from build123d import *

# Parameters (mm, degrees)
SKETCH1_W           = 9
SKETCH1_H           = 9
BOSS_EXTRUDE1_DEPTH = 3
SKETCH2_W           = 2.95
SKETCH2_H           = 6
BOSS_EXTRUDE2_DEPTH = 6.1
FILLET1_R           = 3
SKETCH3_R           = 0.975
CUT_EXTRUDE1_DEPTH  = 11.1
CUT_EXTRUDE3_DEPTH  = 21.1
BOSS_EXTRUDE3_START = 4
SKETCH5_R           = 3
BOSS_EXTRUDE3_DEPTH = 4
SKETCH8_R           = 1.55
CUT_EXTRUDE4_DEPTH  = 3
CUT_EXTRUDE5_DEPTH  = 0.5
SKETCH10_W          = 9
SKETCH10_H          = 3
BOSS_EXTRUDE4_DEPTH = 4
SKETCH11_R          = 1
CUT_EXTRUDE6_DEPTH  = 4
CUT_EXTRUDE7_DEPTH  = 4


with BuildPart() as part:
    # Sketch1 → Boss-Extrude1 (new body)
    with BuildSketch(Plane(origin=(0, 0, 0), x_dir=(1, 0, 0), z_dir=(0, 1, 0))):
        with Locations((4.5, 4.5)):
            Rectangle(SKETCH1_W, SKETCH1_H)
    extrude(amount=BOSS_EXTRUDE1_DEPTH)

    # Sketch2 → Boss-Extrude2 (add)
    with BuildSketch(Plane(origin=(0, 0, -9), x_dir=(-1, 0, 0), z_dir=(0, 0, -1))):
        with Locations((-7.525, 1.5)):
            Rectangle(SKETCH2_W, SKETCH2_H)
        with Locations((-1.475, 1.5)):
            Rectangle(SKETCH2_W, SKETCH2_H)
    extrude(amount=BOSS_EXTRUDE2_DEPTH)

    # Fillet1
    fillet1_edges = [part.edges().sort_by_distance(p)[0] for p in [
        (1.475, 4.5, -15.1),
        (1.475, -1.5, -15.1),
        (7.525, -1.5, -15.1),
        (7.525, 4.5, -15.1),
    ]]
    fillet(fillet1_edges, radius=FILLET1_R - 0.0001)  # a hair under: the kernel refuses the full size

    # Sketch3 → Cut-Extrude1 (cut)
    with BuildSketch(Plane(origin=(9, 0, 0), x_dir=(0, 0, -1), z_dir=(1, 0, 0))):
        with Locations((12.1, 1.5)):
            Circle(SKETCH3_R)
    extrude(amount=-CUT_EXTRUDE1_DEPTH, mode=Mode.SUBTRACT)

    # Sketch6 → Cut-Extrude3 (cut)
    with BuildSketch(Plane.ZY):
        with BuildLine():
            Line((-12.1, 4.5), (-9, 4.5))
            Line((-9, 4.5), (-9, 3))
            Line((-9, 3), (-9.501923789, 3))
            ThreePointArc((-9.501923789, 3), (-10.6, 4.098076211), (-12.1, 4.5))
        make_face()
        with BuildLine():
            Line((-12.1, -1.5), (-9, -1.5))
            Line((-9, -1.5), (-9, 0))
            Line((-9, 0), (-9.501923789, 0))
            ThreePointArc((-9.501923789, 0), (-10.6, -1.098076211), (-12.1, -1.5))
        make_face()
    extrude(amount=-CUT_EXTRUDE3_DEPTH, mode=Mode.SUBTRACT)

    # Sketch5 → Boss-Extrude3 (add)
    with BuildSketch(Plane.ZY.offset(BOSS_EXTRUDE3_START)):
        with Locations((-12.1, 1.5)):
            Circle(SKETCH5_R)
    extrude(amount=-BOSS_EXTRUDE3_DEPTH)

    # Sketch8 → Cut-Extrude4 (cut)
    with BuildSketch(Plane(origin=(0, -1.5, 0), x_dir=(-1, 0, 0), z_dir=(0, -1, 0))):
        with Locations(Location((1.6, 12.1, 0), (0, 0, 90))):
            Circle(SKETCH8_R)
    extrude(amount=-CUT_EXTRUDE4_DEPTH, mode=Mode.SUBTRACT)

    # Sketch9 → Cut-Extrude5 (cut)
    with BuildSketch(Plane.ZY.offset(4)):
        with BuildLine():
            Line((-11.85, 1.5), (-11.85, -0.8))
            ThreePointArc((-11.85, -0.8), (-12.1, -1.05), (-12.35, -0.8))
            Line((-12.35, -0.8), (-12.35, 0.896446609))
            Line((-12.35, 0.896446609), (-13.549568901, -0.303122292))
            ThreePointArc((-13.549568901, -0.303122292), (-13.903122292, -0.303122292), (-13.903122292, 0.050431099))
            Line((-13.903122292, 0.050431099), (-12.703553391, 1.25))
            Line((-12.703553391, 1.25), (-14.4, 1.25))
            ThreePointArc((-14.4, 1.25), (-14.65, 1.5), (-14.4, 1.75))
            Line((-14.4, 1.75), (-12.703553391, 1.75))
            Line((-12.703553391, 1.75), (-13.903122292, 2.949568901))
            ThreePointArc((-13.903122292, 2.949568901), (-13.903122292, 3.303122292), (-13.549568901, 3.303122292))
            Line((-13.549568901, 3.303122292), (-12.35, 2.103553391))
            Line((-12.35, 2.103553391), (-12.35, 3.8))
            ThreePointArc((-12.35, 3.8), (-12.1, 4.05), (-11.85, 3.8))
            Line((-11.85, 3.8), (-11.85, 1.5))
        make_face()
    extrude(amount=-CUT_EXTRUDE5_DEPTH, mode=Mode.SUBTRACT)

    # Sketch10 → Boss-Extrude4 (add)
    with BuildSketch(Plane.XY):
        with Locations((4.5, 1.5)):
            Rectangle(SKETCH10_W, SKETCH10_H)
    extrude(amount=BOSS_EXTRUDE4_DEPTH)

    # Sketch11 → Cut-Extrude6 (cut)
    with BuildSketch(Plane(origin=(0, 3, 0), x_dir=(1, 0, 0), z_dir=(0, 1, 0))):
        with Locations(Location((4.5, -1, 0), (0, 0, 270))):
            Circle(SKETCH11_R)
    extrude(amount=-CUT_EXTRUDE6_DEPTH, mode=Mode.SUBTRACT)

    # Sketch12 → Cut-Extrude7 (cut)
    with BuildSketch(Plane(origin=(0, 3, 0), x_dir=(1, 0, 0), z_dir=(0, 1, 0))):
        with BuildLine():
            add(Edge.make_bspline(
                [(1.5, -1), (1.53988428, 0.555027292), (0.235256098, 1.545486909), (0, 3)],
                knots=[0, 0, 0, 0, 1, 1, 1, 1], degree=3))
            Line((0, 3), (0, -4))
            Line((0, -4), (4.5, -4))
            ThreePointArc((4.5, -4), (2.378679656, -3.121320344), (1.5, -1))
        make_face()
        with BuildLine():
            ThreePointArc((7.5, -1), (6.621320344, -3.121320344), (4.5, -4))
            Line((4.5, -4), (9, -4))
            Line((9, -4), (9, 3))
            add(Edge.make_bspline(
                [(7.5, -1), (7.46011572, 0.555027292), (8.764743902, 1.545486909), (9, 3)],
                knots=[0, 0, 0, 0, 1, 1, 1, 1], degree=3))
        make_face()
    extrude(amount=-CUT_EXTRUDE7_DEPTH, mode=Mode.SUBTRACT)


solid = part.part
Verification items for the finished model (mm, model axes). A direction names the side the tool comes from. Round coordinates to 2 decimals unless told otherwise and drop trailing zeros. Write each loop counter-clockwise with the first axis right and the second up, starting at its lowest first coordinate (ties: lowest second). Pieces come first, ordered by that corner, then holes.
(1) Section check B-B (x = 5.25). Enter the section's corners in (y, z).
Returned:
outline: (0, -9) - (3, -9) - (3, 0.34) - (0, 0.34) - close; (0, 1.66) - (3, 1.66) - (3, 3.9) - (0, 3.9) - close
(2) Material ranges on line 1 (X direction, y = -0.6, z = -12.1); line 2 (Y direction, x = 2.25, z = -12.1) (3 decimals); line 3 (X direction, y = 3.5, z = -10), recorded low to high.
Returned:
line 1: x = -3.5 to -3.15, -0.05 to 2.95, 6.05 to 9
line 2: y = -1.5 to 0.525, 2.475 to 4.5
line 3: x = -4 to 2.95, 6.05 to 9
(3) Access from +Z, -Z, +X, -X, +Y, -Y to the whole of each face (thin tool, end or side, straight path). Record for faces 5 (the cylindrical face through (7.5, 3.64, -14.2)), 6 (the flat face through (4, 0, -4)), 7 (the flat face through (-3.754, 2.341, -13.295)), 8 (the flat face through (4, 1, -9)), 9 (the cylindrical face through (-1.134, -0.021, -13.578)).
Returned:
face 5: -Z, +X, -X, +Y
face 6: +Z, +X, -X, -Y
face 7: -X
face 8: -Z, +Y, -Y
face 9: -Y
(4) Section check A-A (z = 1.5). Enter the section's corners in (x, y).
Returned:
outline: (1.54, 0) - (3.63, 0) - (3.63, 3) - (1.54, 3) - close; (5.37, 0) - (7.46, 0) - (7.46, 3) - (5.37, 3) - close
(5) Depth check by flat-ended pin: pin 1 Ø3 at (x, z) = (-1.6, -12.1) entering from -Y; pin 2 Ø2 at (x, y) = (2.5, 0.5) entering from +Z; pin 3 Ø1.6 at (y, z) = (1.5, -12.1) entering from -X; pin 4 Ø1.6 at (x, z) = (4.5, 1) entering from +Y. Enter the tip coordinate at first touch or a pass-through.
Returned:
pin 1: stops at y = 1.5
pin 2: stops at z = 3.83
pin 3: stops at x = -4
pin 4: passes through
(6) Section check C-C (z = -7). Enter the section's corners in (x, y).
Returned:
outline: (0, 0) - (9, 0) - (9, 3) - (0, 3) - close
(7) Mould release check, pull along Y, two halves, no side actions. Record for faces 1 (the cylindrical face through (7.546, 1.543, -11.126)), 2 (the cylindrical face through (1.45, 3.64, -14.2)), 3 (the flat face through (0, 1, -6)), 4 (the flat face through (0, 2, -12)): pulls with the +Y half, pulls with the -Y half, needs draft (parallel to the pull), parting line crosses it, or undercut.
Returned:
face 1: undercut
face 2: pulls with the +Y half
face 3: needs draft
face 4: undercut
(8) Section check D-D (x = 3.25). Enter the section's corners in (y, z).
Returned:
outline: (0, -9) - (3, -9) - (3, 3.73) - (0, 3.73) - close
